```python
from build123d import *

# Parameters (mm, degrees)
F1_DEPTH  = 15
F3_DEPTH  = 15
F4_DEPTH  = 10
F5_DEPTH  = 15
F6_DEPTH  = 14
F8_DEPTH  = 9
F9_DEPTH  = 11.1596047133
F10_DEPTH = 11.1596047133
F12_DEPTH = 1


with BuildPart() as f1:
    # F0 (on Front) → F1 (new body)
    with BuildSketch(Plane.XZ):
        Polygon((0, 20), (0, 0), (60, 0), (60, 20), (45, 20), (30, 5.0404220819), (15, 20), align=None)
    extrude(amount=-F1_DEPTH)

    # F2 (on face) → F3 (cut, through all)
    with BuildSketch(Plane.XZ):
        Polygon((18.6596047133, 2.4207425304), (22.8898393214, 2.4207425304), (22.8898393214, 8.3013760923), (18.6596047133, 12.520211041), (14.3979182423, 16.770413096), (11.1596047133, 20), (0, 20), (0, 2.4207425304), align=None)
        Polygon((37.1101606786, 2.4207425304), (41.3403952867, 2.4207425304), (60, 2.4207425304), (60, 20), (48.8403952867, 20), (45.6020817577, 16.770413096), (41.3403952867, 12.520211041), (37.1101606786, 8.3013760923), align=None)
    extrude(amount=-F3_DEPTH, mode=Mode.SUBTRACT)

    # F2 (on face) → F4 (cut)
    with BuildSketch(Plane.XZ):
        Polygon((0, 0), (22.8898393214, 0), (22.8898393214, 2.4207425304), (18.6596047133, 2.4207425304), (0, 2.4207425304), align=None)
        Polygon((60, 2.4207425304), (41.3403952867, 2.4207425304), (37.1101606786, 2.4207425304), (37.1101606786, 0), (60, 0), align=None)
    extrude(amount=-F4_DEPTH, mode=Mode.SUBTRACT)

    # F2 (on face) → F5 (join, through all)
    with BuildSketch(Plane.XZ):
        Polygon((45, 20), (48.8403952867, 20), (48.8403952867, 23.5034972429), (15, 23.5034972429), (11.1596047133, 23.5034972429), (11.1596047133, 20), (15, 20), align=None)
    extrude(amount=-F5_DEPTH)

    # F2 (on face) → F6 (cut)
    with BuildSketch(Plane.XZ):
        Polygon((45, 20), (48.8403952867, 20), (48.8403952867, 23.5034972429), (15, 23.5034972429), (11.1596047133, 23.5034972429), (11.1596047133, 20), (15, 20), align=None)
    extrude(amount=-F6_DEPTH, mode=Mode.SUBTRACT)

    # F7 (on face) → F8 (join)
    with BuildSketch(Plane.XZ):
        Polygon((26.9925054163, 0), (29.0075894445, 0), (31.0043748468, 0), (33.0223664641, 0), (33.0223664641, 5.0404220819), (33.0223664641, 8.0546438564), (30, 5.0404220819), (26.9925054163, 8.0398120528), (26.9925054163, 6.030158284), align=None)
    extrude(amount=F8_DEPTH)

    # F9 (cut, through all): a face of the model
    f9_faces = [f1.faces().sort_by_distance(p)[0] for p in [
        (0, 12.5, 1.2103712652),
    ]]
    extrude(f9_faces, amount=-F9_DEPTH, mode=Mode.SUBTRACT)

    # F10 (cut, through all): a face of the model
    f10_faces = [f1.faces().sort_by_distance(p)[0] for p in [
        (60, 12.5, 1.2103712652),
    ]]
    extrude(f10_faces, amount=-F10_DEPTH, mode=Mode.SUBTRACT)

    # F11 (on face) → F12 (join)
    with BuildSketch(Plane.XZ.offset(9)):
        Polygon((33.0223664641, 8.0546438564), (26.9925054163, 8.0398120528), (30, 5.0404220819), align=None)
        Polygon((30, 5.0404220819), (26.9925054163, 8.0398120528), (26.9925054163, 0), (33.0223664641, 0), (33.0223664641, 8.0546438564), align=None)
    extrude(amount=F12_DEPTH)


solid = f1.part
```
Source: CAD feature listing. Evaluate the final solid. Frame: model axes, mm. A direction names the side the tool comes from. Give positions to 0.01 mm unless a question says otherwise; leave off trailing zeros. Loops run counter-clockwise (first coordinate to the right, second up) from the corner with the lowest first, then second, coordinate; pieces in that order, holes last. Notation, with made-up numbers: (5, 29.5) -> (12, 29.5) arc R32 cw to (12, 62.5) -> close; hole circle Ø6 at (20, -30.5). An arc over 180 degrees is marked (long way). Use a Markdown table: item, result. Add a question column.
(1) Section query A-A (x = 46). Output: boundary loops of the cut face in (y, z).
(2) Ray query, line 1 (Z direction, x = 20.5, y = 14.25); line 2 (X direction, y = 12.5, z = 6.25); line 3 (Y direction, x = 43, z = 22). Return the intervals inside material, ascending.
(3) Section query B-B (y = 9.25). Output: boundary loops of the cut face in (x, z), then the cut area to 3 significant figures.
(4) Section query C-C (z = 15). Output: boundary loops of the cut face in (x, y).
(5) Section query D-D (z = 5.75). Output: boundary loops of the cut face in (x, y).
(6) First-contact query: pin 1 Ø4 at (x, z) = (36, 22) entering from -Y; pin 2 Ø2 at (y, z) = (7, 12.5) entering from +X; pin 3 Ø2.5 at (y, z) = (10.5, 6) entering from +X. Flat tips, straight axial feed; report the tip coordinate or a pass-through.
(7) Pull-direction query (Z, two-part tool) for faces 1 (the face through (11.16, 12, 1)), 2 (the face through (43, 12, 2.421)), 3 (the face through (30.3, 14.5, 23.503)); classes: +Z half, -Z half, draft (parallel to the pull), parting line (faces both ways), or undercut.
(8) Access query for faces 4 (the face through (21.4, 0, 10)), 5 (the face through (38.6, 0, 10)), 6 (the face through (43, 10, 1)), 7 (the face through (47, 7, 20)), 8 (the face through (30, -9, 7)). Directions: +Z, -Z, +X, -X, +Y, -Y. A direction counts if a zero-diameter tool reaches every point of the face in a straight line with its end or side. Return the directions, or none.
Checked values:
| question | item | result |
|---|---|---|
| 1 | outline | (0, 17.17) -> (15, 17.17) -> (15, 23.5) -> (14, 23.5) -> (14, 20) -> (0, 20) -> close; (10, 0) -> (15, 0) -> (15, 2.42) -> (10, 2.42) -> close |
| 2 | line 1 | 0 to 2.42, 10.68 to 14.51, 20 to 23.5 |
| 2 | line 2 | 22.89 to 28.79, 31.21 to 37.11 |
| 2 | line 3 | 14 to 15 |
| 3 | outline | (11.16, 20) -> (22.89, 8.3) -> (22.89, 0) -> (37.11, 0) -> (37.11, 8.3) -> (48.84, 20) -> (45, 20) -> (30, 5.04) -> (15, 20) -> close |
| 3 | area | 197 mm^2 |
| 4 | outline | (16.17, 0) -> (20.01, 0) -> (20.01, 15) -> (16.17, 15) -> close; (39.99, 0) -> (43.83, 0) -> (43.83, 15) -> (39.99, 15) -> close |
| 5 | outline | (22.89, 0) -> (26.99, 0) -> (26.99, -10) -> (33.02, -10) -> (33.02, 0) -> (37.11, 0) -> (37.11, 15) -> (30.71, 15) -> (30.71, -9) -> (29.29, -9) -> (29.29, 15) -> (22.89, 15) -> close |
| 6 | pin 1 | y = 14 |
| 6 | pin 2 | x = 42.32 |
| 6 | pin 3 | x = 37.11 |
| 7 | face 1 | draft |
| 7 | face 2 | undercut |
| 7 | face 3 | +Z half |
| 8 | face 4 | +Z, -Z, -X, -Y |
| 8 | face 5 | +Z, -Z, +X, -Y |
| 8 | face 6 | -Z, +X, -Y |
| 8 | face 7 | +Z, +X, -X, -Y |
| 8 | face 8 | +Z, +Y |
